Source: CAD feature listing. Evaluate the final solid. Frame: model axes, mm. A direction names the side the tool comes from. Round coordinates to 2 decimals unless told otherwise and drop trailing zeros. Order: outer loops, then holes, each group sorted by start corner. A loop starts at its lowest first (then second) coordinate and runs counter-clockwise, first axis right, second up. Notation, with made-up numbers: (62.5, 74) -> (74.5, 74) arc R15 ccw to (74.5, 79) -> close; hole circle Ø8 at (49, -23.5). An arc over 180 degrees is marked (long way). Answer as CSV lines item,"result". Start each with the question number.
(1) Contact query for flat-ended pins moving along their axis: P1, Ø1, axis at x = -1.5, z = -6, coming from the +Y side; P2, Ø4, axis at x = 1.5, z = -7, coming from the +Y side; P3, Ø1.5, axis at x = 2.5, y = 2.5, coming from the -Z side. Output: stop coordinate, or through.
(2) Line query: line 1 along Z through (x, y) = (-2.5, 0.75); line 2 along Y through (x, z) = (-1, 3); line 3 along Z through (x, y) = (-0.5, 0.5). Output: solid intervals per line, ascending. Write a range as from..to.
(3) Section query A-A (x = 0). Output: boundary loops of the cut face in (y, z), plus the area to 3 significant figures.
(4) Section query B-B (z = -7). Output: boundary loops of the cut face in (x, y).
(5) Set-up query: faces 4 (the flat face through (0, 1.5, 3)), 5 (the flat face through (-2, 2, 0)), 6 (the cylindrical face through (3.233, 1.341, 1.927)). Return all of +Z, -Z, +X, -X, +Y, -Y with unobstructed straight access to the full face (end or side cutting, diameter ignored); none if empty.
(6) Pull-direction query (Y, two-part tool) for faces 1 (the flat face through (-1.305, -0.74, 3.014)), 2 (the flat face through (0, 0, -12)), 3 (the cylindrical face through (0, 2, -6)); classes: +Y half, -Y half, draft (parallel to the pull), parting line (faces both ways), or undercut.
(7) Section query C-C (z = 0.75). Output: boundary loops of the cut face in (x, y), plus the area to 3 significant figures.
```python
from build123d import *

# Parameters (mm, degrees)
CUT_EXTRUDE1_DEPTH = 2
CHAMFER1_SIZE      = 0.35


with BuildPart() as part:
    # Sketch1 → Revolve1 (revolve)
    with BuildSketch(Plane.XZ, mode=Mode.PRIVATE) as revolve1_sk:
        with BuildLine():
            Line((0, -12), (-2, -12))
            Line((-2, -12), (-2, 0))
            Line((-2, 0), (-3.5, 0))
            Line((-3.5, 0), (-3.5, 3.8))
            ThreePointArc((-3.5, 3.8), (-3.441421356, 3.941421356), (-3.3, 4))
            Line((-3.3, 4), (0, 4))
            Line((0, 4), (0, -12))
        make_face()
    revolve(revolve1_sk.sketch.rotate(Axis((0, 0, 4), (0, 0, -1)), 180), axis=Axis((0, 0, 4), (0, 0, -1)))

    # Sketch2 → Cut-Extrude1 (cut)
    with BuildSketch(Plane.XY.offset(4)):
        Polygon((1.732050808, 0), (0.866025404, 1.5), (-0.866025404, 1.5), (-1.732050808, 0), (-0.866025404, -1.5), (0.866025404, -1.5), align=None)
    extrude(amount=-CUT_EXTRUDE1_DEPTH, mode=Mode.SUBTRACT)

    # Chamfer1
    chamfer1_edges = [part.edges().sort_by_distance(p)[0] for p in [
        (-2, 0, -12),
    ]]
    chamfer(chamfer1_edges, length=CHAMFER1_SIZE)


solid = part.part
```
Answer block:
1,P1,"y = 1.73"
1,P2,"y = 2"
1,P3,"z = 0"
2,line 1,"0..4"
2,line 2,"-3.35..-1.27, 1.27..3.35"
2,line 3,"-12..2"
3,outline,"(-3.5, 0) -> (-2, 0) -> (-2, -11.65) -> (-1.65, -12) -> (1.65, -12) -> (2, -11.65) -> (2, 0) -> (3.5, 0) -> (3.5, 3.8) arc R0.2 ccw to (3.3, 4) -> (1.5, 4) -> (1.5, 2) -> (-1.5, 2) -> (-1.5, 4) -> (-3.3, 4) arc R0.2 ccw to (-3.5, 3.8) -> close"
3,area,"69.9 mm2"
4,outline,"circle Ø4 at (0, 0)"
5,face 4,"+Z"
5,face 5,"-Z"
5,face 6,"+Z, -Z"
6,face 1,"undercut"
6,face 2,"draft"
6,face 3,"parting line"
7,outline,"circle Ø7 at (0, 0)"
7,area,"38.5 mm2"
